from build123d import *

# Parameters (mm, degrees)
ESBO_O1_W                = 300
ESBO_O1_H                = 1300
RESSALTO_EXTRUS_O1_DEPTH = 18
CORTE_EXTRUS_O1_DEPTH    = 668.326007286
ESBO_O3_R                = 37.5
CORTE_EXTRUS_O2_DEPTH    = 668.326007286
CORTE_EXTRUS_O3_DEPTH    = 668.326007286


with BuildPart() as part:
    # Esboço1 → Ressalto-extrusão1 (new body)
    with BuildSketch(Plane.XY):
        Rectangle(ESBO_O1_W, ESBO_O1_H)
    extrude(amount=RESSALTO_EXTRUS_O1_DEPTH)

    # Esboço2 → Corte-extrusão1 (cut, through all)
    with BuildSketch(Plane(origin=(0, 0, 0), x_dir=(-1, 0, 0), z_dir=(0, 0, -1))):
        with BuildLine():
            Line((-80, -650), (80, -650))
            Line((80, -650), (80, -550))
            ThreePointArc((80, -550), (74.142135624, -535.857864376), (60, -530))
            Line((60, -530), (-60, -530))
            ThreePointArc((-60, -530), (-74.142135624, -535.857864376), (-80, -550))
            Line((-80, -550), (-80, -650))
        make_face()
    extrude(amount=-CORTE_EXTRUS_O1_DEPTH, mode=Mode.SUBTRACT)

    # Esboço3 → Corte-extrusão2 (cut, through all)
    with BuildSketch(Plane(origin=(0, 0, 0), x_dir=(-1, 0, 0), z_dir=(0, 0, -1))):
        with Locations((0, 335)):
            Circle(ESBO_O3_R)
    extrude(amount=-CORTE_EXTRUS_O2_DEPTH, mode=Mode.SUBTRACT)

    # Esboço4 → Corte-extrusão3 (cut, through all)
    with BuildSketch(Plane.XY.offset(18)):
        Polygon((-37, 402.517498316), (37, 402.482501684), (37, 426.517498316), (-37, 426.517498316), align=None)
    extrude(amount=-CORTE_EXTRUS_O3_DEPTH, mode=Mode.SUBTRACT)


solid = part.part
The listing builds one solid part. Answer for the finished solid, in the listing's coordinates (mm). Give positions to 0.01 mm unless a question says otherwise; leave off trailing zeros. Order: outer loops, then holes, each group sorted by start corner. A loop starts at its lowest first (then second) coordinate and runs counter-clockwise, first axis right, second up. Notation, with made-up numbers: (38.5, -11.5) - (43.5, -11.5) arc R13 ccw to (43.5, 10.5) - close; hole circle Ø4 at (-16.75, 71.5). An arc over 180 degrees is marked (long way). Use one line per item in the form item = value.
1) Find section B-B on x = 0. Determine the outline of the cut face in (y, z), and give its area (3 significant figures).
Verdict:
outline = (-530, 0) - (297.5, 0) - (297.5, 18) - (-530, 18) - close; (372.5, 0) - (402.5, 0) - (402.5, 18) - (372.5, 18) - close; (426.52, 0) - (650, 0) - (650, 18) - (426.52, 18) - close
area = 19,500 mm^2
2) Find section C-C on z = 11.75. Determine the outline of the cut face in (x, y).
Verdict:
outline = (-150, -650) - (-80, -650) - (-80, -550) arc R20 cw to (-60, -530) - (60, -530) arc R20 cw to (80, -550) - (80, -650) - (150, -650) - (150, 650) - (-150, 650) - close; hole circle Ø75 at (0, 335); hole (-37, 402.52) - (37, 402.48) - (37, 426.52) - (-37, 426.52) - close
3) Consider probe 1 along Y at (x, z) = (0, 10); probe 2 along X at (y, z) = (329, 6); probe 3 along Y at (x, z) = (5, 16.5). Determine where each line is inside the solid, lowest interval first. Write a range as [from, to].
Verdict:
probe_1 = [-530, 297.5], [372.5, 402.5], [426.52, 650]
probe_2 = [-150, -37.02], [37.02, 150]
probe_3 = [-530, 297.83], [372.17, 402.5], [426.52, 650]
4) Each of these flat-tipped pins is pushed along its axis until it touches: pin 1 (9 mm diameter, centred on x = 12, z = 8.5, fed in from -Y); pin 2 (6 mm diameter, centred on x = -96.5, y = 310.5, fed in from -Z). Where does it stop, or does it pass through?
Verdict:
pin_1 = -530
pin_2 = 0
5) The mould has two halves that part along Y. Classify faces 1 (the cylindrical face through (8.13, 298.39, 8.87)), 2 (the flat face through (-2, 9, 0)): released by +Y, released by -Y, zero draft, split by the parting line, or undercut.
Verdict:
face_1 = undercut
face_2 = zero draft
6) Find section A-A on y = 335. Determine the outline of the cut face in (x, z), and give its area (3 significant figures).
Verdict:
outline = (-150, 0) - (-37.5, 0) - (-37.5, 18) - (-150, 18) - close; (37.5, 0) - (150, 0) - (150, 18) - (37.5, 18) - close
area = 4,050 mm^2
